Here's how the part is built. I have some questions about the finished solid (model axes, mm). Coordinates: 2 decimals unless noted, no trailing zeros. Write each loop counter-clockwise with the first axis right and the second up, starting at its lowest first coordinate (ties: lowest second). Pieces come first, ordered by that corner, then holes. Notation, with made-up numbers: (53.25, 11) -> (83.25, 11) arc R28 ccw to (83.25, 43) -> close; hole circle Ø4 at (65, 1.5). An arc over 180 degrees is marked (long way). Put each result on its own line as item: value. Start each with the question number.
Item 1: For pin 1 (2.5 mm diameter, centred on x = -53.13, y = 50.27, fed in from +Z), with a flat end and sliding along its axis, tell me the tip position at first contact or that it passes through.
Item 2: I need wall thicknesses on line 1 (Y direction, x = 4.87, z = 0.45); line 2 (Y direction, x = -52, z = 0.15); line 3 (X direction, y = 51, z = 0.4). Which ranges of each line are inside material? Lowest first, please. Write a range as [from, to].
Item 3: I want a section at A-A, the plane x = -53.13. List the corners of the cut face in (y, z) for me, then the cut area to 3 significant figures.
Item 4: I want a section at B-B, the plane y = 50.27. List the corners of the cut face in (x, z) for me, then the cut area to 3 significant figures.
Autodesk Inventor part; units mm, degrees
ref_plane "YZ Plane" through (0, 0, 0) normal (1, 0, 0) x (0, 1, 0)
ref_plane "XZ Plane" through (0, 0, 0) normal (0, 1, 0) x (-1, 0, 0)
ref_plane "XY Plane" through (0, 0, 0) normal (0, 0, 1) x (1, 0, 0)
sketch "Эскиз1" plane through (0, 0, 0) normal (0, 0, 1) x (1, 0, 0)
  line L0 (-73.63, -2.23) -> (5.37, -2.23)
  arc A0 (5.37, -2.23) -> (8.37, 0.77) centre (5.37, 0.77) ccw
  line L1 (8.37, 0.77) -> (8.37, 50.77)
  arc A1 (8.37, 50.77) -> (5.37, 53.77) centre (5.37, 50.77) ccw
  line L2 (5.37, 53.77) -> (-73.63, 53.77)
  arc A2 (-73.63, 53.77) -> (-76.63, 50.77) centre (-73.63, 50.77) ccw
  line L3 (-76.63, 50.77) -> (-76.63, 0.77)
  arc A3 (-76.63, 0.77) -> (-73.63, -2.23) centre (-73.63, 0.77) ccw
  circle A4 centre (4.87, 50.27) radius 1.35
  circle A5 centre (-53.13, 50.27) radius 1.35
  circle A6 centre (0.07, 48.67) radius 0.325
  circle A7 centre (-5.73, 48.67) radius 0.325
  circle A8 centre (-68.88, 49.235) radius 1.65
  circle A9 centre (4.87, 44.27) radius 1.55
  circle A10 centre (-68.88, 37.805) radius 1.65
  circle A11 centre (-53.13, 7.27) radius 1.55
  circle A12 centre (4.87, 1.27) radius 1.35
  circle A13 centre (-53.13, 1.27) radius 1.35
  line L4 (5.37, -2.23) -> (8.37, -2.23) construction
  line L5 (8.37, -2.23) -> (8.37, 0.77) construction
  line L6 (8.37, 0.77) -> (5.37, 0.77) construction
  line L7 (5.37, 0.77) -> (5.37, -2.23) construction
  line L8 (8.37, -2.23) -> (-56.63, -2.23)
  line L9 (-56.63, -2.23) -> (-56.63, 53.77)
  line L10 (-56.63, 53.77) -> (8.37, 53.77)
  line L11 (8.37, 53.77) -> (8.37, -2.23)
  line L12 (8.37, -2.23) -> (-56.63, -2.23)
  line L13 (-56.63, -2.23) -> (-56.63, -13.23)
  line L14 (-56.63, -13.23) -> (8.37, -13.23)
  line L15 (8.37, -13.23) -> (8.37, -2.23)
  line L16 (-56.63, 53.77) -> (8.37, 53.77)
  line L17 (8.37, 53.77) -> (8.37, 61.77)
  line L18 (8.37, 61.77) -> (-56.63, 61.77)
  line L19 (-56.63, 61.77) -> (-56.63, 53.77)
  point P0 (0, 0)
  point P1 (8.37, 0.77)
  point P2 (8.37, 53.77)
  dimension "d0" = 65
  dimension "d1" = 56
  dimension "d8" = 65
  dimension "d9" = 11
  dimension "d10" = 8
extrude "Выдавливание1" add sketch "Эскиз1" along normal blind 1.5 contours L9 L2 A1 L1 A0 L0 | A0 L11 L8 | L10 L11 A1 | A6 | A7 | A9 | A11
properties part number "board_rpi"
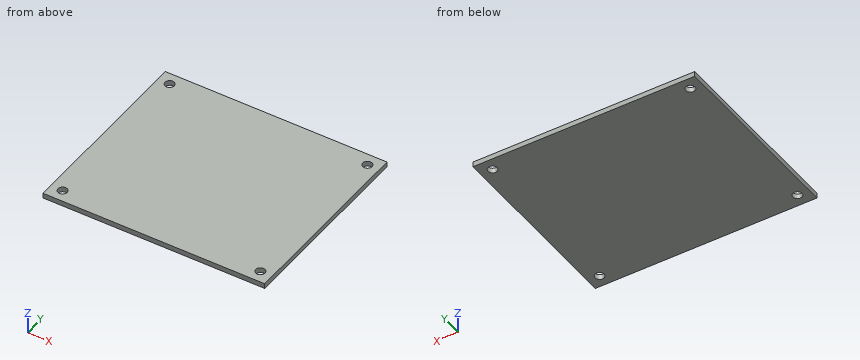
Calculated:
1. pin 1: passes through
2. line 1: y = [-2.23, -0.08], [2.62, 48.92], [51.62, 53.77]
2. line 2: y = [-2.23, 0.53], [2.01, 49.53], [51.01, 53.77]
2. line 3: x = [-56.63, -54.27], [-51.99, 3.73], [6.01, 8.37]
3. outline: (-2.23, 0) -> (-0.08, 0) -> (-0.08, 1.5) -> (-2.23, 1.5) -> close; (2.62, 0) -> (48.92, 0) -> (48.92, 1.5) -> (2.62, 1.5) -> close; (51.62, 0) -> (53.77, 0) -> (53.77, 1.5) -> (51.62, 1.5) -> close
3. area: 75.9 mm2
4. outline: (-56.63, 0) -> (-54.48, 0) -> (-54.48, 1.5) -> (-56.63, 1.5) -> close; (-51.78, 0) -> (3.52, 0) -> (3.52, 1.5) -> (-51.78, 1.5) -> close; (6.22, 0) -> (8.37, 0) -> (8.37, 1.5) -> (6.22, 1.5) -> close
4. area: 89.4 mm2
